Verification items for the finished model (mm, model axes). Give positions to 0.01 mm unless a question says otherwise; leave off trailing zeros. Write each loop counter-clockwise with the first axis right and the second up, starting at its lowest first coordinate (ties: lowest second). Pieces come first, ordered by that corner, then holes. Notation, with made-up numbers: (13, -10.5) - (47, -10.5) arc R19 cw to (47, 10.5) - close; hole circle Ø9 at (51.25, 14). An arc over 180 degrees is marked (long way). Answer as a JSON object with one key per item and string values. Group by question number.
Item 1: Sectioned sample at A-A, the plane y = -124.46. Record the boundary of the cut face in (x, z) (3 decimals), and give its area (3 significant figures).
Item 2: Scan line: line 1 along X through (y, z) = (-71, 6.5). Record every from-to range of solid material in increasing order. Write a range as [from, to].
Item 3: Sectioned sample at D-D, the plane y = -325. Record the boundary of the cut face in (x, z).
Item 4: Sectioned sample at C-C, the plane x = 6.5. Record the boundary of the cut face in (y, z).
Item 5: Go/stop test with flat-tipped pins: pin 1 (25 mm diameter, centred on y = 124.46, z = 0, fed in from +X); pin 2 (5 mm diameter, centred on x = 15.5, z = 1, fed in from -Y). Record where each tip stops, or that it passes through.
Item 6: Sectioned sample at B-B, the plane z = 0. Record the boundary of the cut face in (x, y) (3 decimals), and give its area (3 significant figures).
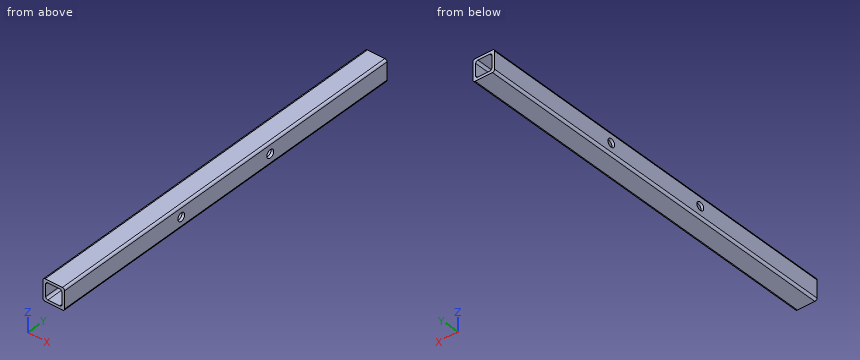
```python
from build123d import *

# Parameters (mm, degrees)
F0_W     = 50.8
F0_H     = 50.8
F0_W_2   = 38.1
F0_H_2   = 38.1
F1_DEPTH = 450.85
F2_R     = 9.525
F3_DEPTH = 50.801
F4_R     = 5.08


with BuildPart() as f1:
    # F0 (on Front) → F1 (new body, symmetric)
    with BuildSketch(Plane.XZ):
        Rectangle(F0_W, F0_H)
        Rectangle(F0_W_2, F0_H_2, mode=Mode.SUBTRACT)
    extrude(amount=F1_DEPTH, both=True)

    # F2 (on face) → F3 (cut, through all)
    with BuildSketch(Plane.YZ.offset(25.4)):
        with Locations((-124.46, 0)):
            Circle(F2_R)
        with Locations((124.46, 0)):
            Circle(F2_R)
    extrude(amount=-F3_DEPTH, mode=Mode.SUBTRACT)

    # F4
    f4_edges = [f1.edges().sort_by_distance(p)[0] for p in [
        (-25.4, 0, 25.4),
        (25.4, 0, 25.4),
        (19.05, 0, -19.05),
        (-19.05, 0, -19.05),
        (-25.4, 0, -25.4),
        (25.4, 0, -25.4),
        (19.05, 0, 19.05),
        (-19.05, 0, 19.05),
    ]]
    fillet(f4_edges, radius=F4_R)


solid = f1.part
```
Geometry check:
{
 "1": {"outline": "(-25.4, -20.32) arc R5.08 ccw to (-20.32, -25.4) - (20.32, -25.4) arc R5.08 ccw to (25.4, -20.32) - (25.4, -9.525) - (19.05, -9.525) - (19.05, -13.97) arc R5.08 cw to (13.97, -19.05) - (-13.97, -19.05) arc R5.08 cw to (-19.05, -13.97) - (-19.05, -9.525) - (-25.4, -9.525) - close; (-25.4, 9.525) - (-19.05, 9.525) - (-19.05, 13.97) arc R5.08 cw to (-13.97, 19.05) - (13.97, 19.05) arc R5.08 cw to (19.05, 13.97) - (19.05, 9.525) - (25.4, 9.525) - (25.4, 20.32) arc R5.08 ccw to (20.32, 25.4) - (-20.32, 25.4) arc R5.08 ccw to (-25.4, 20.32) - close", "area": "887 mm^2"},
 "2": {"line 1": "[-25.4, -19.05], [19.05, 25.4]"},
 "3": {"outline": "(-25.4, -20.32) arc R5.08 ccw to (-20.32, -25.4) - (20.32, -25.4) arc R5.08 ccw to (25.4, -20.32) - (25.4, 20.32) arc R5.08 ccw to (20.32, 25.4) - (-20.32, 25.4) arc R5.08 ccw to (-25.4, 20.32) - close; hole (-19.05, -13.97) arc R5.08 ccw to (-13.97, -19.05) - (13.97, -19.05) arc R5.08 ccw to (19.05, -13.97) - (19.05, 13.97) arc R5.08 ccw to (13.97, 19.05) - (-13.97, 19.05) arc R5.08 ccw to (-19.05, 13.97) - close"},
 "4": {"outline": "(-450.85, -25.4) - (450.85, -25.4) - (450.85, -19.05) - (-450.85, -19.05) - close; (-450.85, 19.05) - (450.85, 19.05) - (450.85, 25.4) - (-450.85, 25.4) - close"},
 "5": {"pin 1": "x = 25.4", "pin 2": "through"},
 "6": {"outline": "(-25.4, -450.85) - (-19.05, -450.85) - (-19.05, -133.985) - (-25.4, -133.985) - close; (-25.4, -114.935) - (-19.05, -114.935) - (-19.05, 114.935) - (-25.4, 114.935) - close; (-25.4, 133.985) - (-19.05, 133.985) - (-19.05, 450.85) - (-25.4, 450.85) - close; (19.05, -450.85) - (25.4, -450.85) - (25.4, -133.985) - (19.05, -133.985) - close; (19.05, -114.935) - (25.4, -114.935) - (25.4, 114.935) - (19.05, 114.935) - close; (19.05, 133.985) - (25.4, 133.985) - (25.4, 450.85) - (19.05, 450.85) - close", "area": "11,000 mm^2"}
}
